from build123d import *

# Parameters (mm, degrees)
F0_R          = 90
F0_R_2        = 70
F1_DEPTH      = 20
F1_DEPTH_BACK = 20
F0_R_3        = 15
F2_DEPTH      = 10
F2_DEPTH_BACK = 10


with BuildPart() as f1:
    # F0 (on Front) → F1 (new body, two sides)
    with BuildSketch(Plane.XZ) as f1_sk:
        with Locations((-22.680921, 0)):
            Circle(F0_R)
        with Locations((-22.680921, 0)):
            Circle(F0_R_2, mode=Mode.SUBTRACT)
    extrude(amount=F1_DEPTH)
    extrude(f1_sk.sketch, amount=-F1_DEPTH_BACK)

    # F0 (on Front) → F2 (join, two sides)
    with BuildSketch(Plane.XZ) as f2_sk:
        with Locations((-22.680921, 0)):
            Circle(F0_R_2)
        with Locations((-22.680921, 0)):
            Circle(F0_R_3, mode=Mode.SUBTRACT)
    extrude(amount=F2_DEPTH)
    extrude(f2_sk.sketch, amount=-F2_DEPTH_BACK)


solid = f1.part
Read the model definition and answer for the solid it produces. Units are mm, in the model's axes. A direction names the side the tool comes from. Give positions to 0.01 mm unless a question says otherwise; leave off trailing zeros. Write each loop counter-clockwise with the first axis right and the second up, starting at its lowest first coordinate (ties: lowest second). Pieces come first, ordered by that corner, then holes. Notation, with made-up numbers: M 84.5,-37.75 L 111.5,-37.75 A20 cw 111.5,-18.75 Z; hole C 86,-7 d4. An arc over 180 degrees is marked long. One line per item, written item: value. Start each with the question number.
(1) Find section C-C (y = 13). Determine the outline of the cut face in (x, z).
(2) Find section B-B (x = -23). Determine the outline of the cut face in (y, z).
(3) A tool of negligible diameter and unlimited length cuts with its end or side. For faces 4 (the flat face through (-24, 10, 17)), 5 (the flat face through (24, -20, -53)), 6 (the flat face through (-24, -10, 17)), from which of +Z, -Z, +X, -X, +Y, -Y can it reach the whole face along a straight path? Write none if from no direction.
(4) Determine the mould class of faces 1 (the cylindrical face through (9.62, 14.93, -62.1)), 2 (the cylindrical face through (-42.19, -0.28, -87.86)), 3 (the flat face through (24, 20, -53)) for opening direction X: pulls with the +X half, pulls with the -X half, needs draft (parallel to the pull), parting line crosses it, or undercut.
(5) Find section D-D (z = -31.5). Determine the outline of the cut face in (x, y).
(6) Flat-ended cylindrical pins translate along their axes: pin 1 Ø8 at (y, z) = (-13.5, -12) entering from +X; pin 2 Ø12 at (y, z) = (-7.5, 63) entering from +X; pin 3 Ø12 at (x, z) = (-11, 55) entering from -Y. Find the tip coordinate at first contact, or state that the pin passes through.
(7) Find the intervals of material crossed by line 1 (Y direction, x = 4, z = 16); line 2 (X direction, y = 14.5, z = 8); line 3 (Z direction, x = 30.5, y = 11.5), in increasing order.
(8) Find section A-A (z = 0). Determine the outline of the cut face in (x, y), plus the area to 3 significant figures.
Results below:
1. outline: C -22.68,0 d180; hole C -22.68,0 d140
2. outline: M -20,-90 L 20,-90 L 20,-70 L 10,-70 L 10,-15 L -10,-15 L -10,-70 L -20,-70 Z; M -20,70 L -10,70 L -10,15 L 10,15 L 10,70 L 20,70 L 20,90 L -20,90 Z
3. face 4: +Y
3. face 5: +Z, -Z, +X, -X, -Y
3. face 6: -Y
4. face 1: undercut
4. face 2: parting line crosses it
4. face 3: needs draft
5. outline: M -106.99,-20 L -85.19,-20 L -85.19,-10 L 39.83,-10 L 39.83,-20 L 61.63,-20 L 61.63,20 L 39.83,20 L 39.83,10 L -85.19,10 L -85.19,20 L -106.99,20 Z
6. pin 1: stops at x = 66.96
6. pin 2: stops at x = 46.97
6. pin 3: stops at y = -10
7. line 1: y = -10 to 10
7. line 2: x = -112.32 to -92.22, 46.86 to 66.96
7. line 3: z = -72.61 to -45.52, 45.52 to 72.61
8. outline: M -112.68,-20 L -92.68,-20 L -92.68,-10 L -37.68,-10 L -37.68,10 L -92.68,10 L -92.68,20 L -112.68,20 Z; M -7.68,-10 L 47.32,-10 L 47.32,-20 L 67.32,-20 L 67.32,20 L 47.32,20 L 47.32,10 L -7.68,10 Z
8. area: 3,800 mm^2
